Geometry check sheet. Reference: the model listing, model coordinates, mm. A direction names the side the tool comes from. Round coordinates to 2 decimals unless told otherwise and drop trailing zeros. Order: outer loops, then holes, each group sorted by start corner. A loop starts at its lowest first (then second) coordinate and runs counter-clockwise, first axis right, second up. Notation, with made-up numbers: (-36, 87.25) -> (-9, 87.25) arc R25 ccw to (-9, 117.25) -> close; hole circle Ø6 at (3, -14). An arc over 180 degrees is marked (long way). Use a Markdown table: item, result. Add a question column.
Item 1: Gauge pin test, flat ends, axial feed: pin 1 Ø6 at (y, z) = (13.5, -2) entering from +X (3 decimals); pin 2 Ø6 at (x, z) = (10.5, -6) entering from +Y (3 decimals). Record the tip position at first contact, or that the pin passes through.
Item 2: Material ranges on probe 1 along Z at (x, y) = (12.7, 1.25); probe 2 along Y at (x, z) = (1.8, -6.35); probe 3 along X at (y, z) = (0.9, -6.35), recorded low to high. Write a range as [from, to].
Item 3: Mould release check, pull along Z, two halves, no side actions. Record for faces 1 (the flat face through (14, 3.175, 0)), 2 (the cylindrical face through (14.8, 1.57, 7.69)), 3 (the flat face through (8, 3, -12.7)): pulls with the +Z half, pulls with the -Z half, needs draft (parallel to the pull), parting line crosses it, or undercut.
Item 4: Sectioned sample at B-B, the plane x = 12.7. Record the cut outline in (y, z) (3 decimals).
Item 5: Sectioned sample at A-A, the plane z = -6.35. Record the cut outline in (x, y) (3 decimals), and give its area (3 significant figures).
Item 6: Sectioned sample at C-C, the plane z = 2. Record the cut outline in (x, y) (3 decimals).
Item 7: Sectioned sample at D-D, the plane y = 15.75. Record the cut outline in (x, z) (3 decimals).
Item 8: Set-up check for faces 4 (the flat face through (8, 3, 12.7)), 5 (the flat face through (3.175, 11, 0)): record each of +Z, -Z, +X, -X, +Y, -Y from which the full face is reachable in a straight line by a thin tool's end or side.
from build123d import *

# Parameters (mm, degrees)
BOSS_EXTRUDE1_DEPTH     = 12.7
CUT_EXTRUDE1_DEPTH      = 33.534068682
CUT_EXTRUDE1_DEPTH_BACK = 33.534068682
SKETCH3_R               = 2.4892
CUT_EXTRUDE2_DEPTH      = 32.908355097
CUT_EXTRUDE2_DEPTH_BACK = 32.908355097
SKETCH4_R               = 2.4892


with BuildPart() as part:
    # Sketch1 → Boss-Extrude1 (new, symmetric)
    with BuildSketch(Plane.XY):
        Polygon((0, 0), (0, 19.05), (3.175, 19.05), (3.175, 3.175), (25.4, 3.175), (25.4, 0), align=None)
    extrude(amount=BOSS_EXTRUDE1_DEPTH, both=True)

    # Sketch3 → Cut-Extrude1 (cut, two sides: drawn at the far end of the back side and taken through both)
    with BuildSketch(Plane(origin=(0, 3.175, 0), x_dir=(1, 0, 0), z_dir=(0, 1, 0)).offset(-CUT_EXTRUDE1_DEPTH_BACK)):
        with Locations(Location((12.7, -6.35, 0), (0, 0, 270))):
            Circle(SKETCH3_R)
        with Locations(Location((12.7, 6.35, 0), (0, 0, 270))):
            Circle(SKETCH3_R)
    extrude(amount=CUT_EXTRUDE1_DEPTH + CUT_EXTRUDE1_DEPTH_BACK, mode=Mode.SUBTRACT)

    # Sketch4 → Cut-Extrude2 (cut, two sides: drawn at the far end of the back side and taken through both)
    with BuildSketch(Plane(origin=(3.175, 0, 0), x_dir=(0, 0, -1), z_dir=(1, 0, 0)).offset(-CUT_EXTRUDE2_DEPTH_BACK)):
        with Locations(Location((-6.35, 12.7, 0), (0, 0, 90))):
            Circle(SKETCH4_R)
        with Locations(Location((6.35, 12.7, 0), (0, 0, 90))):
            Circle(SKETCH4_R)
    extrude(amount=CUT_EXTRUDE2_DEPTH + CUT_EXTRUDE2_DEPTH_BACK, mode=Mode.SUBTRACT)


solid = part.part
Found:
| question | item | result |
|---|---|---|
| 1 | pin 1 | stops at x = 3.175 |
| 1 | pin 2 | stops at y = 3.175 |
| 2 | probe 1 | z = [-12.7, -8.84], [-3.86, 3.86], [8.84, 12.7] |
| 2 | probe 2 | y = [0, 10.21], [15.19, 19.05] |
| 2 | probe 3 | x = [0, 10.21], [15.19, 25.4] |
| 3 | face 1 | needs draft |
| 3 | face 2 | undercut |
| 3 | face 3 | pulls with the -Z half |
| 4 | outline | (0, -12.7) -> (3.175, -12.7) -> (3.175, -8.839) -> (0, -8.839) -> close; (0, -3.861) -> (3.175, -3.861) -> (3.175, 3.861) -> (0, 3.861) -> close; (0, 8.839) -> (3.175, 8.839) -> (3.175, 12.7) -> (0, 12.7) -> close |
| 5 | outline | (0, 0) -> (10.211, 0) -> (10.211, 3.175) -> (3.175, 3.175) -> (3.175, 10.211) -> (0, 10.211) -> close; (0, 15.189) -> (3.175, 15.189) -> (3.175, 19.05) -> (0, 19.05) -> close; (15.189, 0) -> (25.4, 0) -> (25.4, 3.175) -> (15.189, 3.175) -> close |
| 5 | area | 99.4 mm2 |
| 6 | outline | (0, 0) -> (25.4, 0) -> (25.4, 3.175) -> (3.175, 3.175) -> (3.175, 19.05) -> (0, 19.05) -> close |
| 7 | outline | (0, -12.7) -> (3.175, -12.7) -> (3.175, 12.7) -> (0, 12.7) -> close |
| 8 | face 4 | +Z, +X, -X, +Y, -Y |
| 8 | face 5 | +Z, -Z, +X, +Y |
